Geometry check sheet. Reference: drawing and pictorial views, mm from the part's lowest x, y, z. A direction names the side the tool comes from. Coordinates: 2 decimals unless noted, no trailing zeros. Write each loop counter-clockwise with the first axis right and the second up, starting at its lowest first coordinate (ties: lowest second). Pieces come first, ordered by that corner, then holes. Notation, with made-up numbers: (-13.5, -28.5) -> (20.5, -28.5) arc R16 cw to (20.5, -22.5) -> close; hole circle Ø11 at (24.25, 89). An arc over 180 degrees is marked (long way). Answer in a Markdown table with one row per item.
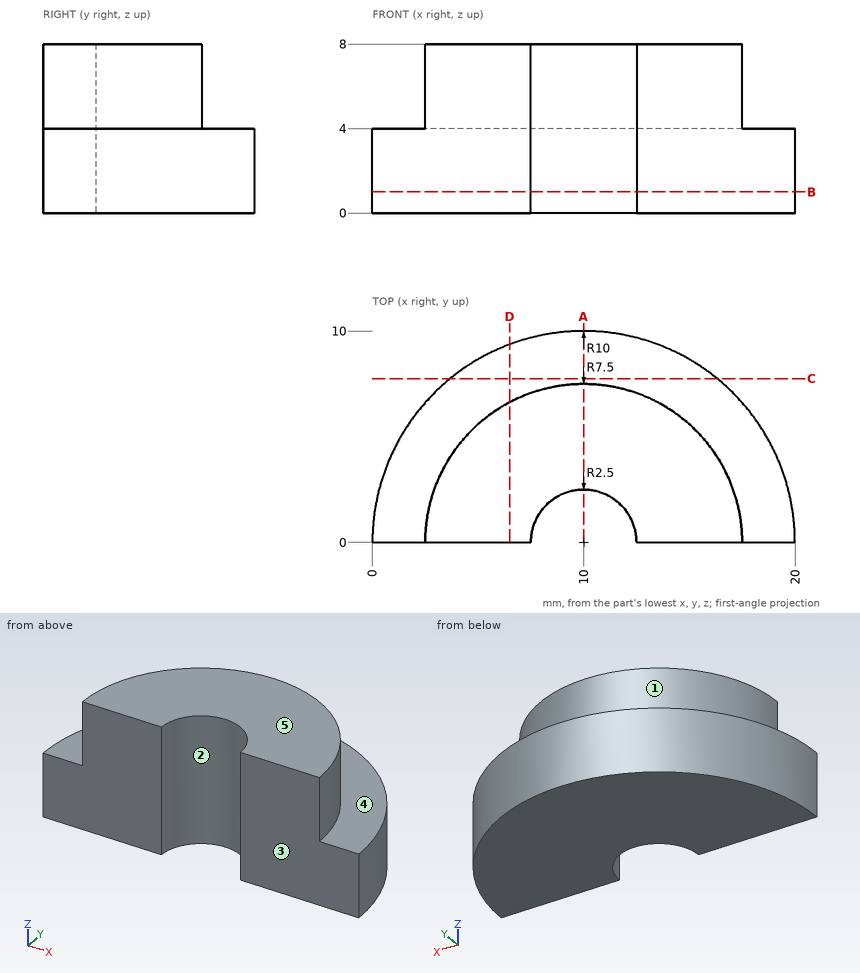
1. Section check C-C, the plane y = 7.75. Record the boundary of the cut face in (x, z).
Geometry says:
| item | result |
|---|---|
| outline | (3.68, 0) -> (16.32, 0) -> (16.32, 4) -> (3.68, 4) -> close |
2. Tool access check on the marked faces 4 and 5. Record the directions out of +Z, -Z, +X, -X, +Y, -Y that give a thin tool (end or side, any length) a straight path to the whole face; none if there is none.
Geometry says:
| item | result |
|---|---|
| face 4 | +Z, +Y |
| face 5 | +Z, +X, -X, +Y, -Y |
3. Thickness scan on line 1 (X direction, y = 2.25, z = 7.25); line 2 (Y direction, x = 10, z = 1.5); line 3 (X direction, y = 1.25, z = 5). Record the ranges inside material, lowest first. Write a range as from..to.
Geometry says:
| item | result |
|---|---|
| line 1 | 2.85..8.91, 11.09..17.15 |
| line 2 | 2.5..10 |
| line 3 | 2.6..7.83, 12.17..17.4 |
4. Depth check by flat-ended pin: P1, Ø3, axis at x = 3, z = 2.5, coming from the +Y side; P2, Ø4, axis at y = 9, z = 4.5, coming from the -X side; P3, Ø1.5, axis at x = 7.5, y = 2, coming from the -Z side; P4, Ø4, axis at x = 6, z = 5, coming from the +Y side. Enter the tip coordinate at first touch or a pass-through.
Geometry says:
| item | result |
|---|---|
| P1 | y = 8.35 |
| P2 | x = 2.92 |
| P3 | z = 0 |
| P4 | y = 9.74 |
5. Section check A-A, the plane x = 10. Record the boundary of the cut face in (y, z), plus the area to 3 significant figures.
Geometry says:
| item | result |
|---|---|
| outline | (2.5, 0) -> (10, 0) -> (10, 4) -> (7.5, 4) -> (7.5, 8) -> (2.5, 8) -> close |
| area | 50.0 mm^2 |
6. Mould release check, pull along X, two halves, no side actions. Record for the marked faces 1, 2 and 3: released by +X, released by -X, zero draft, split by the parting line, or undercut.
Geometry says:
| item | result |
|---|---|
| face 1 | split by the parting line |
| face 2 | undercut |
| face 3 | zero draft |
7. Section check D-D, the plane x = 6.5. Record the boundary of the cut face in (y, z).
Geometry says:
| item | result |
|---|---|
| outline | (0, 0) -> (9.37, 0) -> (9.37, 4) -> (6.63, 4) -> (6.63, 8) -> (0, 8) -> close |
8. Section check B-B, the plane z = 1. Record the boundary of the cut face in (x, y).
Geometry says:
| item | result |
|---|---|
| outline | (0, 0) -> (7.5, 0) arc R2.5 cw to (12.5, 0) -> (20, 0) arc R10 ccw to start |
